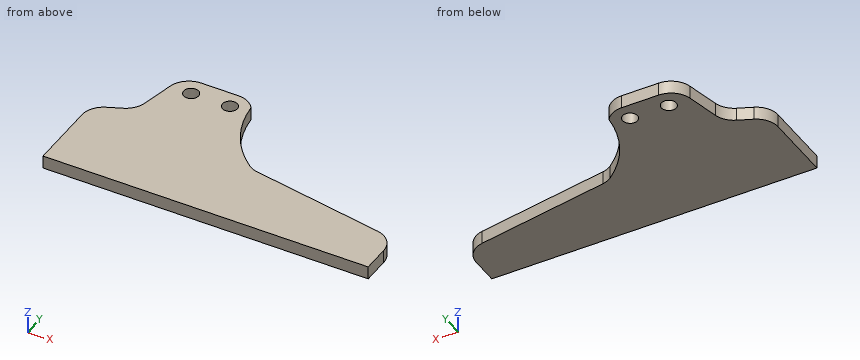
from build123d import *

# Parameters (mm, degrees)
CROQUIS2_R              = 3.435535485
SALIENTE_EXTRUIR1_DEPTH = 6


with BuildPart() as part:
    # Croquis2 → Saliente-Extruir1 (new body)
    with BuildSketch(Plane.XY):
        with BuildLine():
            Line((75.476244536, -42.362655144), (-74.410975533, -42.362655144))
            Line((-74.410975533, -42.362655144), (-74.410975533, -10.730962139))
            ThreePointArc((-74.410975533, -10.730962139), (-72.792282586, -5.276267639), (-68.460237116, -1.587468243))
            Line((-68.460237116, -1.587468243), (-62.049591399, 1.251532003))
            ThreePointArc((-62.049591399, 1.251532003), (-58.348209926, 4.076202257), (-56.327089342, 8.270729457))
            Line((-56.327089342, 8.270729457), (-53.063252273, 23.284379976))
            ThreePointArc((-53.063252273, 23.284379976), (-49.529087977, 29.006996787), (-43.186320825, 31.244845149))
            Line((-43.186320825, 31.244845149), (-26.148431061, 31.244845149))
            ThreePointArc((-26.148431061, 31.244845149), (-21.368566285, 30.043227891), (-17.725183812, 26.724078081))
            ThreePointArc((-17.725183812, 26.724078081), (-11.921972825, 7.766213541), (1.029468531, -7.245050647))
            ThreePointArc((1.029468531, -7.245050647), (3.120257187, -8.473650696), (5.443510228, -9.168884899))
            Line((5.443510228, -9.168884899), (67.083811667, -19.782734484))
            ThreePointArc((67.083811667, -19.782734484), (73.098451393, -23.231181656), (75.476244536, -29.743767833))
            Line((75.476244536, -29.743767833), (75.476244536, -42.362655144))
        make_face()
        with Locations((-25.582237715, 23.471115745)):
            Circle(CROQUIS2_R, mode=Mode.SUBTRACT)
        with Locations((-43.316057918, 23.228186701)):
            Circle(CROQUIS2_R, mode=Mode.SUBTRACT)
    extrude(amount=SALIENTE_EXTRUIR1_DEPTH)


solid = part.part
Read the model definition and answer for the solid it produces. Units are mm, in the model's axes. Round coordinates to 2 decimals unless told otherwise and drop trailing zeros. Loops run counter-clockwise (first coordinate to the right, second up) from the corner with the lowest first, then second, coordinate; pieces in that order, holes last. Notation, with made-up numbers: (42, 7.25) - (91, 7.25) arc R20 ccw to (91, 44.25) - close; hole circle Ø11 at (-9, 23). An arc over 180 degrees is marked (long way). One line per question, with ' | ' between items. Start each with the question number.
Q1. Flat-ended cylindrical pins translate along their axes: pin 1 (1 mm diameter, centred on y = 18, z = 3, fed in from +X); pin 2 (1 mm diameter, centred on x = 16.5, z = 3, fed in from +Y); pin 3 (2 mm diameter, centred on y = 22.5, z = 1.5, fed in from +X) (3 decimals). Find the tip coordinate at first contact, or state that the pin passes through.
Q2. Section A-A on z = 2.65 is taken. Give the vertices of the cut face in (x, y).
Q3. Find the intervals of material crossed by L1, parallel to X at y = 8.5, z = 2.7; L2, parallel to X at y = 6.5, z = 0.6; L3, parallel to Y at x = 17.5, z = 4.9, in increasing order.
Q4. Section C-C on x = 46.5 is taken. Give the vertices of the cut face in (y, z), plus the area to 3 significant figures.
Q5. Section B-B on x = 15 is taken. Give the vertices of the cut face in (y, z), plus the area to 3 significant figures.
Established:
1) pin 1: x = -15.98 | pin 2: y = -10.99 | pin 3: x = -16.965
2) outline: (-74.41, -42.36) - (75.48, -42.36) - (75.48, -29.74) arc R10.11 ccw to (67.08, -19.78) - (5.44, -9.17) arc R10.11 cw to (1.03, -7.25) arc R48.14 cw to (-17.73, 26.72) arc R10.11 ccw to (-26.15, 31.24) - (-43.19, 31.24) arc R10.11 ccw to (-53.06, 23.28) - (-56.33, 8.27) arc R10 cw to (-62.05, 1.25) - (-68.46, -1.59) arc R10 ccw to (-74.41, -10.73) - close; hole circle Ø6.87 at (-43.32, 23.23); hole circle Ø6.87 at (-25.58, 23.47)
3) L1: -56.28 to -12.32 | L2: -56.89 to -11.2 | L3: -42.36 to -11.24
4) outline: (-42.36, 0) - (-16.24, 0) - (-16.24, 6) - (-42.36, 6) - close | area: 157 mm²
5) outline: (-42.36, 0) - (-10.81, 0) - (-10.81, 6) - (-42.36, 6) - close | area: 189 mm²
